from build123d import *

# Parameters (mm, degrees)
SKETCH_1_R                      = 4
EXTRUDE_1_DEPTH                 = 15
SKETCH_4_W                      = 59.231964801
SKETCH_4_H                      = 71.825442386
CUT_EXTRUDE_3_DEPTH             = 5
SKETCH_5_R                      = 5
SKETCH_5_R_2                    = 2.5
CUT_EXTRUDE_1_DEPTH             = 109.069666358
CHAMFER_1_SIZE                  = 10
CHAMFER_2_SIZE                  = 7.5
CHAMFER_2_SIZE2                 = 10.967511122
FILLET_1_R                      = 5
SKETCH_6_R                      = 2
CUT_EXTRUDE_2_DEPTH             = 109.069666358
SKETCH_7_R                      = 3
CUT_EXTRUDE_3_2_DEPTH           = 1.5
CUT_EXTRUDE_3_2_DRAFT           = -33
CUT_EXTRUDE_3_2_PROFILE_2_DEPTH = 1.5
CUT_EXTRUDE_3_2_PROFILE_2_DRAFT = -33
CUT_EXTRUDE_3_2_PROFILE_3_DEPTH = 1.5
CUT_EXTRUDE_3_2_PROFILE_3_DRAFT = -33
CUT_EXTRUDE_3_2_PROFILE_4_DEPTH = 1.5
CUT_EXTRUDE_3_2_PROFILE_4_DRAFT = -33
CUT_EXTRUDE_3_2_PROFILE_5_DEPTH = 1.5
CUT_EXTRUDE_3_2_PROFILE_5_DRAFT = -33
CUT_EXTRUDE_3_2_PROFILE_6_DEPTH = 1.5
CUT_EXTRUDE_3_2_PROFILE_6_DRAFT = -33
CHAMFER_3_SIZE                  = 3


with BuildPart() as part:
    # Эскиз1 → Вытянуть1 (new body)
    with BuildSketch(Plane(origin=(0, 0, 0), x_dir=(0, 0, -1), z_dir=(1, 0, 0))):
        Polygon((-24.582546576, -0.000617064), (-24.582546576, -32.845704832), (-6.76628281, -32.845704832), (-6.76628281, -98.258905102), (33.827639979, -98.258905102), (42.417453424, -61.027347877), (42.417453424, -0.000617064), align=None)
        with Locations((13.620132913, -77.029686591)):
            Circle(SKETCH_1_R, mode=Mode.SUBTRACT)
    extrude(amount=EXTRUDE_1_DEPTH)

    # Эскиз4 → Cut-Extrude 3 (cut)
    with BuildSketch(Plane.ZY):
        with Locations((-12.801471023, -76.114894855)):
            Rectangle(SKETCH_4_W, SKETCH_4_H)
    extrude(amount=-CUT_EXTRUDE_3_DEPTH, mode=Mode.SUBTRACT)

    # Эскиз5 → Вырез-Вытянуть1 (cut, through all)
    with BuildSketch(Plane(origin=(15, 0, 0), x_dir=(0, 0, -1), z_dir=(1, 0, 0))):
        with Locations((-9.068801992, -16.42316095)):
            Circle(SKETCH_5_R)
        with Locations((24.417453448, -16.423160953)):
            Circle(SKETCH_5_R_2)
        with Locations((37.417453448, -16.423160948)):
            Circle(SKETCH_5_R_2)
    extrude(amount=-CUT_EXTRUDE_1_DEPTH, mode=Mode.SUBTRACT)

    # Фаска1
    chamfer_1_edges = [part.edges().sort_by_distance(p)[0] for p in [
        (10, -98.258905102, 6.76628281),
    ]]
    chamfer(chamfer_1_edges, length=CHAMFER_1_SIZE)

    # Фаска2
    chamfer_2_edges = [part.edges().sort_by_distance(p)[0] for p in [
        (10, -98.258905102, -33.827639979),
    ]]
    chamfer_2_side = [part.faces().sort_by_distance(p)[0] for p in [
        (10, -98.258905102, -18.530678584),
    ]]
    chamfer(chamfer_2_edges, length=CHAMFER_2_SIZE, length2=CHAMFER_2_SIZE2, reference=chamfer_2_side[0])

    # Скругление1
    fillet_1_edges = [part.edges().sort_by_distance(p)[0] for p in [
        (7.5, -32.845704832, 6.76628281),
    ]]
    fillet(fillet_1_edges, radius=FILLET_1_R)

    # Эскиз6 → Вырез-Вытянуть2 (cut, through all)
    with BuildSketch(Plane(origin=(15, 0, 0), x_dir=(0, 0, -1), z_dir=(1, 0, 0))):
        with Locations((-16.16411161, -6.276498114)):
            Circle(SKETCH_6_R)
        with Locations((8.83588839, -6.276498105)):
            Circle(SKETCH_6_R)
        with Locations((33.83588839, -6.276498095)):
            Circle(SKETCH_6_R)
        with Locations((-16.164111603, -26.569823822)):
            Circle(SKETCH_6_R)
        with Locations((8.835888397, -26.569823813)):
            Circle(SKETCH_6_R)
        with Locations((33.835888397, -26.569823803)):
            Circle(SKETCH_6_R)
    extrude(amount=-CUT_EXTRUDE_2_DEPTH, mode=Mode.SUBTRACT)


with BuildPart() as cut_extrude_3_2_tool:
    # Эскиз7 → Cut-Extrude 3 2 (with draft: the straight prism first)
    with BuildSketch(Plane(origin=(15, 0, 0), x_dir=(0, 0, -1), z_dir=(1, 0, 0))):
        with Locations((-16.16411161, -6.276498114)):
            Circle(SKETCH_7_R)
    extrude(amount=-CUT_EXTRUDE_3_2_DEPTH)
    # Cut-Extrude 3 2: the draft: its side faces are tilted about the plane it starts from
    cut_extrude_3_2_sides = [cut_extrude_3_2_tool.faces().sort_by_distance(p)[0] for p in [
        (14.25, -6.276498114, 19.16411161),
    ]]
    draft(cut_extrude_3_2_sides, Plane(origin=(15, 0, 0), x_dir=(0, 0, -1), z_dir=(1, 0, 0)), CUT_EXTRUDE_3_2_DRAFT)


with BuildPart() as part_1:
    add(part.part)

    # Cut-Extrude 3 2: cut by cut_extrude_3_2_tool
    add(cut_extrude_3_2_tool.part, mode=Mode.SUBTRACT)


with BuildPart() as cut_extrude_3_2_profile_2_tool:
    # Эскиз7 → Cut-Extrude 3 2 profile 2 (with draft: the straight prism first)
    with BuildSketch(Plane(origin=(15, 0, 0), x_dir=(0, 0, -1), z_dir=(1, 0, 0))):
        with Locations((8.83588839, -6.276498105)):
            Circle(SKETCH_7_R)
    extrude(amount=-CUT_EXTRUDE_3_2_PROFILE_2_DEPTH)
    # Cut-Extrude 3 2 profile 2: the draft: its side faces are tilted about the plane it starts from
    cut_extrude_3_2_profile_2_sides = [cut_extrude_3_2_profile_2_tool.faces().sort_by_distance(p)[0] for p in [
        (14.25, -6.276498105, -5.83588839),
    ]]
    draft(cut_extrude_3_2_profile_2_sides, Plane(origin=(15, 0, 0), x_dir=(0, 0, -1), z_dir=(1, 0, 0)), CUT_EXTRUDE_3_2_PROFILE_2_DRAFT)


with BuildPart() as part_2:
    add(part_1.part)

    # Cut-Extrude 3 2 profile 2: cut by cut_extrude_3_2_profile_2_tool
    add(cut_extrude_3_2_profile_2_tool.part, mode=Mode.SUBTRACT)


with BuildPart() as cut_extrude_3_2_profile_3_tool:
    # Эскиз7 → Cut-Extrude 3 2 profile 3 (with draft: the straight prism first)
    with BuildSketch(Plane(origin=(15, 0, 0), x_dir=(0, 0, -1), z_dir=(1, 0, 0))):
        with Locations((33.83588839, -6.276498095)):
            Circle(SKETCH_7_R)
    extrude(amount=-CUT_EXTRUDE_3_2_PROFILE_3_DEPTH)
    # Cut-Extrude 3 2 profile 3: the draft: its side faces are tilted about the plane it starts from
    cut_extrude_3_2_profile_3_sides = [cut_extrude_3_2_profile_3_tool.faces().sort_by_distance(p)[0] for p in [
        (14.25, -6.276498095, -30.83588839),
    ]]
    draft(cut_extrude_3_2_profile_3_sides, Plane(origin=(15, 0, 0), x_dir=(0, 0, -1), z_dir=(1, 0, 0)), CUT_EXTRUDE_3_2_PROFILE_3_DRAFT)


with BuildPart() as part_3:
    add(part_2.part)

    # Cut-Extrude 3 2 profile 3: cut by cut_extrude_3_2_profile_3_tool
    add(cut_extrude_3_2_profile_3_tool.part, mode=Mode.SUBTRACT)


with BuildPart() as cut_extrude_3_2_profile_4_tool:
    # Эскиз7 → Cut-Extrude 3 2 profile 4 (with draft: the straight prism first)
    with BuildSketch(Plane(origin=(15, 0, 0), x_dir=(0, 0, -1), z_dir=(1, 0, 0))):
        with Locations((-16.164111603, -26.569823822)):
            Circle(SKETCH_7_R)
    extrude(amount=-CUT_EXTRUDE_3_2_PROFILE_4_DEPTH)
    # Cut-Extrude 3 2 profile 4: the draft: its side faces are tilted about the plane it starts from
    cut_extrude_3_2_profile_4_sides = [cut_extrude_3_2_profile_4_tool.faces().sort_by_distance(p)[0] for p in [
        (14.25, -26.569823822, 19.164111603),
    ]]
    draft(cut_extrude_3_2_profile_4_sides, Plane(origin=(15, 0, 0), x_dir=(0, 0, -1), z_dir=(1, 0, 0)), CUT_EXTRUDE_3_2_PROFILE_4_DRAFT)


with BuildPart() as part_4:
    add(part_3.part)

    # Cut-Extrude 3 2 profile 4: cut by cut_extrude_3_2_profile_4_tool
    add(cut_extrude_3_2_profile_4_tool.part, mode=Mode.SUBTRACT)


with BuildPart() as cut_extrude_3_2_profile_5_tool:
    # Эскиз7 → Cut-Extrude 3 2 profile 5 (with draft: the straight prism first)
    with BuildSketch(Plane(origin=(15, 0, 0), x_dir=(0, 0, -1), z_dir=(1, 0, 0))):
        with Locations((8.835888397, -26.569823813)):
            Circle(SKETCH_7_R)
    extrude(amount=-CUT_EXTRUDE_3_2_PROFILE_5_DEPTH)
    # Cut-Extrude 3 2 profile 5: the draft: its side faces are tilted about the plane it starts from
    cut_extrude_3_2_profile_5_sides = [cut_extrude_3_2_profile_5_tool.faces().sort_by_distance(p)[0] for p in [
        (14.25, -26.569823813, -5.835888397),
    ]]
    draft(cut_extrude_3_2_profile_5_sides, Plane(origin=(15, 0, 0), x_dir=(0, 0, -1), z_dir=(1, 0, 0)), CUT_EXTRUDE_3_2_PROFILE_5_DRAFT)


with BuildPart() as part_5:
    add(part_4.part)

    # Cut-Extrude 3 2 profile 5: cut by cut_extrude_3_2_profile_5_tool
    add(cut_extrude_3_2_profile_5_tool.part, mode=Mode.SUBTRACT)


with BuildPart() as cut_extrude_3_2_profile_6_tool:
    # Эскиз7 → Cut-Extrude 3 2 profile 6 (with draft: the straight prism first)
    with BuildSketch(Plane(origin=(15, 0, 0), x_dir=(0, 0, -1), z_dir=(1, 0, 0))):
        with Locations((33.835888397, -26.569823803)):
            Circle(SKETCH_7_R)
    extrude(amount=-CUT_EXTRUDE_3_2_PROFILE_6_DEPTH)
    # Cut-Extrude 3 2 profile 6: the draft: its side faces are tilted about the plane it starts from
    cut_extrude_3_2_profile_6_sides = [cut_extrude_3_2_profile_6_tool.faces().sort_by_distance(p)[0] for p in [
        (14.25, -26.569823803, -30.835888397),
    ]]
    draft(cut_extrude_3_2_profile_6_sides, Plane(origin=(15, 0, 0), x_dir=(0, 0, -1), z_dir=(1, 0, 0)), CUT_EXTRUDE_3_2_PROFILE_6_DRAFT)


with BuildPart() as part_6:
    add(part_5.part)

    # Cut-Extrude 3 2 profile 6: cut by cut_extrude_3_2_profile_6_tool
    add(cut_extrude_3_2_profile_6_tool.part, mode=Mode.SUBTRACT)

    # Фаска3
    chamfer_3_edges = [part_6.edges().sort_by_distance(p)[0] for p in [
        (15, -0.000617064, -8.917453424),
    ]]
    chamfer(chamfer_3_edges, length=CHAMFER_3_SIZE)


solid = part_6.part
Can you work these out from the model? Positions are in its coordinate system, mm. A direction names the side the tool comes from. Coordinates: 2 decimals unless noted, no trailing zeros. Order: outer loops, then holes, each group sorted by start corner. A loop starts at its lowest first (then second) coordinate and runs counter-clockwise, first axis right, second up. Notation, with made-up numbers: M 51.25,-37 L 62.25,-37 A8 ccw 62.25,-22 Z; hole C -20.5,-6.75 d4. An arc over 180 degrees is marked long. Answer as CSV lines item,"result".
(1) Suppose I cut it at B-B on x = 3.75. Count the separate pieces of the cut face and the enclosed holes in it, plus the area to 3 significant figures.
Geometry check:
separate pieces,"1"
enclosed holes,"9"
area,"2,370 mm^2"
(2) On a 3-axis mill with a long thin cutter (end or side, diameter ignored), from which of +Z, -Z, +X, -X, +Y, -Y can I reach the whole of each face in a straight line? I mean faces 1 (the flat face through (7, -32.846, 18)), 2 (the flat face through (2, -40.202, -18)), 3 (the flat face through (7, -16, 24.583)). Say none if no direction works.
Geometry check:
face 1,"+Z, +X, -X, -Y"
face 2,"+Z, -Z, -X, -Y"
face 3,"+Z, +X, -X, +Y, -Y"
(3) I'm going to push flat-ended pins straight in: pin 1 (8 mm diameter, centred on y = -79, z = -18, fed in from -X); pin 2 (3 mm diameter, centred on y = -5.5, z = -9, fed in from +X); pin 3 (2.5 mm diameter, centred on x = 2, z = -28, fed in from -Y). Where does each tip first touch, or does it pass through?
Geometry check:
pin 1,"x = 5"
pin 2,"x = 13.91"
pin 3,"y = -40.2"
(4) Please list where these lines run through material, in increasing order: L1, parallel to Z at x = 8.25, y = -6.5; L2, parallel to Z at x = 13.5, y = -7.5; L3, parallel to Y at x = 5.5, z = -8.5.
Geometry check:
L1,"-42.42 to -35.82, -31.85 to -10.82, -6.85 to 14.18, 18.15 to 24.58"
L2,"-42.42 to -35.45, -32.22 to -10.45, -7.22 to 14.55, 17.78 to 24.58"
L3,"-98.26 to -28.54, -24.6 to -8.25, -4.3 to 0"
(5) If we mould it in two halves opening along Y, with no side actions, what happens to faces 4 (the flat face through (6, -0.001, -9)), 5 (the cylindrical face through (9.93, -80.578, -15.466)), 6 (the flat face through (5, -69, -18))? For each: released by +Y, released by -Y, zero draft, split by the parting line, or undercut.
Geometry check:
face 4,"released by +Y"
face 5,"undercut"
face 6,"zero draft"
(6) Suppose I cut it at D-D on z = -16. Please give me the cut outline in (x, y), plus the area to 3 significant figures.
Geometry check:
outline,"M 0,-40.2 L 5,-40.2 L 5,-73.81 L 15,-73.81 L 15,-3 L 12,0 L 0,0 Z; M 5,-98.26 L 15,-98.26 L 15,-80.24 L 5,-80.24 Z"
area,"1,110 mm^2"
(7) Suppose I cut it at A-A on z = 8.5. Please give me the cut outline in (x, y), plus the area to 3 significant figures.
Geometry check:
outline,"M 0,-34.06 L 15,-34.06 L 15,-21.39 L 0,-21.39 Z; M 0,-11.46 L 15,-11.46 L 15,-3 L 12,0 L 0,0 Z"
area,"357 mm^2"
